```python
from build123d import *

# Parameters (mm, degrees)
SKETCH_1_R          = 4.9
EXTRUDE_1_DEPTH     = 3
SKETCH_2_R          = 1.6
CUT_EXTRUDE_1_DEPTH = 8.551158851
CHAMFER_1_SIZE      = 1.2
FILLET_1_R          = 1
FILLET_2_R          = 1


with BuildPart() as part:
    # 草图1 → 凸台-拉伸1 (new body)
    with BuildSketch(Plane.XY):
        Circle(SKETCH_1_R)
    extrude(amount=EXTRUDE_1_DEPTH)

    # 草图2 → 切除-拉伸1 (cut, through all)
    with BuildSketch(Plane.XY.offset(3)):
        Circle(SKETCH_2_R)
    extrude(amount=-CUT_EXTRUDE_1_DEPTH, mode=Mode.SUBTRACT)

    # 倒角1
    chamfer_1_edges = [part.edges().sort_by_distance(p)[0] for p in [
        (-1.6, 0, 3),
    ]]
    chamfer(chamfer_1_edges, length=CHAMFER_1_SIZE)

    # 圆角1
    fillet_1_edges = [part.edges().sort_by_distance(p)[0] for p in [
        (-4.9, 0, 3),
    ]]
    fillet(fillet_1_edges, radius=FILLET_1_R)

    # 圆角2
    fillet_2_edges = [part.edges().sort_by_distance(p)[0] for p in [
        (-4.9, 0, 0),
    ]]
    fillet(fillet_2_edges, radius=FILLET_2_R)


solid = part.part
```
Can you work these out from the model? Positions are in its coordinate system, mm. Coordinates: 2 decimals unless noted, no trailing zeros. Loops run counter-clockwise (first coordinate to the right, second up) from the corner with the lowest first, then second, coordinate; pieces in that order, holes last. Notation, with made-up numbers: (-2.5, -2.75) - (38.5, -2.75) arc R13 cw to (38.5, 20.25) - close; hole circle Ø7 at (-14, 63.25). An arc over 180 degrees is marked (long way). Use a Markdown table: item, result.
Item 1: I want a section at A-A on y = 0. Please give me the cut outline in (x, z).
Numbers:
| item | result |
|---|---|
| outline | (-4.9, 1) arc R1 ccw to (-3.9, 0) - (-1.6, 0) - (-1.6, 1.8) - (-2.8, 3) - (-3.9, 3) arc R1 ccw to (-4.9, 2) - close; (1.6, 0) - (3.9, 0) arc R1 ccw to (4.9, 1) - (4.9, 2) arc R1 ccw to (3.9, 3) - (2.8, 3) - (1.6, 1.8) - close |
Item 2: Will these pins go through, and if not, where does the flat tip stop? pin 1 (5 mm diameter, centred on x = 0.5, y = 1, fed in from +Z); pin 2 (3.5 mm diameter, centred on x = 0, y = 0, fed in from +Z); pin 3 (1.5 mm diameter, centred on y = 1.5, z = 2, fed in from +X); pin 4 (1 mm diameter, centred on y = 2, z = 0.5, fed in from +X).
Numbers:
| item | result |
|---|---|
| pin 1 | stops at z = 3 |
| pin 2 | stops at z = 1.95 |
| pin 3 | stops at x = 4.84 |
| pin 4 | stops at x = 4.61 |
Item 3: We'd pull the mould along X, two halves only. Please class faces 1 (the face through (-1.062, -4.783, 1.493)), 2 (the face through (0, -2, 0)), 3 (the face through (-1.27, -0.97, 0.91)): released by +X, released by -X, zero draft, split by the parting line, or undercut.
Numbers:
| item | result |
|---|---|
| face 1 | split by the parting line |
| face 2 | zero draft |
| face 3 | undercut |
Item 4: I want a section at C-C on z = 0.7. Please give me the cut outline in (x, y).
Numbers:
| item | result |
|---|---|
| outline | circle Ø9.71 at (0, 0); hole circle Ø3.2 at (0, 0) |
Item 5: If I drill on probe 1 along Y at (x, z) = (0, 1.3); probe 2 along Y at (x, z) = (-0.25, 0.5); probe 3 along X at (y, z) = (1.25, 2.1), over which ranges is the centre line in solid material (lowest first)? Write a range as from..to.
Numbers:
| item | result |
|---|---|
| probe 1 | y = -4.9..-1.6, 1.6..4.9 |
| probe 2 | y = -4.76..-1.58, 1.58..4.76 |
| probe 3 | x = -4.73..-1.43, 1.43..4.73 |
